from build123d import *

# Parameters (mm, degrees)
F0_W     = 114.3
F0_H     = 101.6
F1_DEPTH = 25.4
F2_W     = 25.4
F2_H     = 12.7
F3_DEPTH = 25.4
F7_D     = 10.16


# Not quite as in the source:
# - a feature of the source that left no trace in its solid (it failed there, or was rolled back) is left out


with BuildPart() as f1:
    # F0 (on Front) → F1 (new body)
    with BuildSketch(Plane.XZ):
        with Locations((-44.2425758362, 44.6146523613)):
            Rectangle(F0_W, F0_H)
    extrude(amount=F1_DEPTH)

    # F2 (on face) → F3 (join)
    with BuildSketch(Plane.XY.offset(95.4146523613)):
        with Locations((0.2074241638, 6.35)):
            Rectangle(F2_W, F2_H)
    extrude(amount=-F3_DEPTH)

    # F5: union 

    # F7 (through all)
    with Locations(Plane.XY.offset(95.4146523613)):
        with Locations((0.2074241638, 6.35)):
            Hole(F7_D / 2)


solid = f1.part
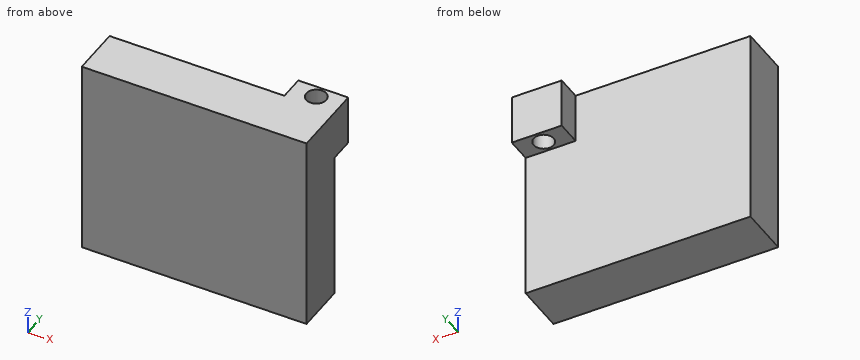
Read the model definition and answer for the solid it produces. Units are mm, in the model's axes. Round coordinates to 2 decimals unless told otherwise and drop trailing zeros. Order: outer loops, then holes, each group sorted by start corner. A loop starts at its lowest first (then second) coordinate and runs counter-clockwise, first axis right, second up. Notation, with made-up numbers: (81, 35.5) - (116, 35.5) arc R32 cw to (116, 61.5) - close; hole circle Ø2 at (63.25, 41.25). An arc over 180 degrees is marked (long way). Use one line per item in the form item = value. Start each with the question number.
(1) Find the intervals of material crossed by line 1 along Y through (x, z) = (-77.5, 70); line 2 along Y through (x, z) = (1.5, 86.5), in increasing order. Write a range as from..to.
(2) The part is cut by section A-A (y = 6.35). Give the vertices of the cut face in (x, z), then the cut area to 3 significant figures.
(3) The part is cut by section C-C (x = -44.5). Give the vertices of the cut face in (y, z), then the cut area to 3 significant figures.
(4) The part is cut by section B-B (z = 81). Give the vertices of the cut face in (x, y).
(5) The part is cut by section D-D (z = 19). Give the vertices of the cut face in (x, y), then the cut area to 3 significant figures.
(6) Flat-ended cylindrical pins translate along their axes: pin 1 Ø4 at (x, z) = (-54.5, 47) entering from +Y; pin 2 Ø14 at (y, z) = (9, 83) entering from -X; pin 3 Ø6.5 at (x, y) = (1.5, 5) entering from -Z; pin 4 Ø10 at (y, z) = (8.5, 5) entering from -X. Find the tip coordinate at first contact, or state that the pin passes through.
Checked values:
q1.line_1 = -25.4..0
q1.line_2 = -25.4..1.44, 11.26..12.7
q2.outline = (-12.49, 70.01) - (-4.87, 70.01) - (-4.87, 95.41) - (-12.49, 95.41) - close; (5.29, 70.01) - (12.91, 70.01) - (12.91, 95.41) - (5.29, 95.41) - close
q2.area = 387 mm^2
q3.outline = (-25.4, -6.19) - (0, -6.19) - (0, 95.41) - (-25.4, 95.41) - close
q3.area = 2,580 mm^2
q4.outline = (-101.39, -25.4) - (12.91, -25.4) - (12.91, 12.7) - (-12.49, 12.7) - (-12.49, 0) - (-101.39, 0) - close; hole circle Ø10.16 at (0.21, 6.35)
q5.outline = (-101.39, -25.4) - (12.91, -25.4) - (12.91, 0) - (-101.39, 0) - close
q5.area = 2,900 mm^2
q6.pin_1 = 0
q6.pin_2 = -12.49
q6.pin_3 = 70.01
q6.pin_4 = through
